from build123d import *

# Parameters (mm, degrees)
SKETCH1_R           = 3
SKETCH1_R_2         = 2
SKETCH1_R_3         = 1.5
BOSS_EXTRUDE1_DEPTH = 5


with BuildPart() as part:
    # Sketch1 → Boss-Extrude1 (new body)
    with BuildSketch(Plane.XY):
        with BuildLine():
            Line((7.589765397, 12.5), (20, 12.5))
            Line((20, 12.5), (20, 5))
            Line((20, 5), (26, 5))
            Line((26, 5), (26, -5))
            Line((26, -5), (20, -5))
            Line((20, -5), (20, -12.5))
            Line((20, -12.5), (0, -12.5))
            Line((0, -12.5), (-22, -12.5))
            ThreePointArc((-22, -12.5), (-24.121320344, -11.621320344), (-25, -9.5))
            Line((-25, -9.5), (-25, 0.5))
            ThreePointArc((-25, 0.5), (-25.465496735, 2.105083549), (-26.717528799, 3.212059663))
            ThreePointArc((-26.717528799, 3.212059663), (-30.169638016, 4.962862371), (-33.519694565, 6.901802618))
            Line((-33.519694565, 6.901802618), (-42.934572397, 12.704217168))
            ThreePointArc((-42.934572397, 12.704217168), (-43.687123123, 12.564740135), (-44.120631689, 11.933981258))
            Line((-44.120631689, 11.933981258), (-44.388558942, 10.673482635))
            ThreePointArc((-44.388558942, 10.673482635), (-45.031133401, 9.939380171), (-45.993109182, 10.101894657))
            ThreePointArc((-45.993109182, 10.101894657), (-52.796527237, 13.506575009), (-60.398778904, 13.796601081))
            ThreePointArc((-60.398778904, 13.796601081), (-61.546162789, 13.706067739), (-62.68972312, 13.836282296))
            Line((-62.68972312, 13.836282296), (-64.396986027, 14.199172229))
            ThreePointArc((-64.396986027, 14.199172229), (-65.658503782, 15.066189361), (-65.937457847, 16.571290812))
            Line((-65.937457847, 16.571290812), (-65.463517392, 18.801005349))
            ThreePointArc((-65.463517392, 18.801005349), (-64.892317345, 20.370364581), (-63.91067059, 21.721485427))
            Line((-63.91067059, 21.721485427), (-62.501386729, 23.180841584))
            ThreePointArc((-62.501386729, 23.180841584), (-59.939578156, 24.750719897), (-56.937877783, 24.881776966))
            Line((-56.937877783, 24.881776966), (-40.62810218, 21.415027142))
            Line((-40.62810218, 21.415027142), (-7.413387902, 14.126720197))
            ThreePointArc((-7.413387902, 14.126720197), (0.044223211, 12.90786831), (7.589765397, 12.5))
        make_face()
        with Locations((10, 0)):
            Circle(SKETCH1_R, mode=Mode.SUBTRACT)
        with Locations((-19.2, -5.8)):
            Circle(SKETCH1_R_2, mode=Mode.SUBTRACT)
        with Locations((-54.590724376, 18.248830539)):
            Circle(SKETCH1_R_3, mode=Mode.SUBTRACT)
        with Locations((-44.809248369, 16.169713631)):
            Circle(SKETCH1_R_3, mode=Mode.SUBTRACT)
    extrude(amount=BOSS_EXTRUDE1_DEPTH)


solid = part.part
The listing builds one solid part. Answer for the finished solid, in the listing's coordinates (mm). A direction names the side the tool comes from. Give positions to 0.01 mm unless a question says otherwise; leave off trailing zeros. Write each loop counter-clockwise with the first axis right and the second up, starting at its lowest first coordinate (ties: lowest second). Pieces come first, ordered by that corner, then holes.
1) Find the intervals of material crossed by L1, parallel to Y at x = 10, z = 2.8; L2, parallel to X at y = -7, z = 1.15; L3, parallel to Y at x = 15.5, z = 2.45, in increasing order.
2) Section C-C (z = 3.1) is taken. Count the separate pieces of the cut face and the enclosed holes in it, and give its area (3 significant figures).
3) Section D-D (x = -52) is taken. Write down the section's boundary in (y, z), and give its area (3 significant figures).
4) For a pull along Y with two mould halves and no side action, classify faces 3 (the face through (23, -5, 2)), 4 (the face through (20, -9, 2)), 5 (the face through (12.77, -1.15, 2.46)), 6 (the face through (-59.98, 24.74, 2.46)) as pulls with the +Y half, pulls with the -Y half, needs draft (parallel to the pull), parting line crosses it, or undercut.
5) Section B-B (x = 10) is taken. Write down the section's boundary in (y, z).
6) Given P1, Ø2, axis at y = 12, z = 1.5, coming from the +X side; P2, Ø1.5, axis at y = -4, z = 2, coming from the -X side; P3, Ø1.5, axis at x = 22.5, z = 3, coming from the -Y side, each flat-ended and moving along its own axis, determine where each tip first touches the part or whether it passes through.
7) Section A-A (y = -5.8) is taken. Write down the section's boundary in (x, z).
8) A tool of negligible diameter and unlimited length cuts with its end or side. For faces 1 (the face through (-25, -5, 2)), 2 (the face through (26, 0, 2)), from which of +Z, -Z, +X, -X, +Y, -Y can it reach the whole face along a straight path? Write none if from no direction.
Response:
1. L1: y = -12.5 to -3, 3 to 12.5
1. L2: x = -25 to -20.8, -17.6 to 20
1. L3: y = -12.5 to 12.5
2. separate pieces: 1
2. enclosed holes: 4
2. area: 1,660 mm2
3. outline: (13.28, 0) - (23.83, 0) - (23.83, 5) - (13.28, 5) - close
3. area: 52.7 mm2
4. face 3: pulls with the -Y half
4. face 4: needs draft
4. face 5: undercut
4. face 6: pulls with the +Y half
5. outline: (-12.5, 0) - (-3, 0) - (-3, 5) - (-12.5, 5) - close; (3, 0) - (12.5, 0) - (12.5, 5) - (3, 5) - close
6. P1: stops at x = 20
6. P2: stops at x = -25
6. P3: stops at y = -5
7. outline: (-25, 0) - (-21.2, 0) - (-21.2, 5) - (-25, 5) - close; (-17.2, 0) - (20, 0) - (20, 5) - (-17.2, 5) - close
8. face 1: +Z, -Z, -X, -Y
8. face 2: +Z, -Z, +X, +Y, -Y
